from build123d import *

# Parameters (mm, degrees)
F1_DEPTH = 40


# Not quite as in the source:
# - ends of sketch curves that miss each other by under 0.0002 mm in the source are joined


with BuildPart() as f1:
    # F0 (on Front) → F1 (new body)
    with BuildSketch(Plane.XZ):
        with BuildLine():
            Line((-4.9999998882, 0), (0, 0))
            Line((0, 0), (0, 370))
            ThreePointArc((0, 370), (-25, 395), (-50, 370))
            Line((-50, 370), (-247.7872705737, 399.6680905861))
            Line((-247.7872705737, 399.6680905861), (-248.5289721923, 394.7234131282))
            Line((-248.5289721923, 394.7234131282), (-50, 364.9440672994))
            Line((-50, 364.9440672994), (-45, 364.9440672994))
            Line((-45, 364.9440672994), (-45, 370))
            ThreePointArc((-45, 370), (-25, 390), (-5, 370))
            Line((-5, 370), (-4.9999998882, 0))
        make_face()
    extrude(amount=-F1_DEPTH)


solid = f1.part
Source: CAD feature listing. Evaluate the final solid. Frame: model axes, mm. Give positions to 0.01 mm unless a question says otherwise; leave off trailing zeros. Loops run counter-clockwise (first coordinate to the right, second up) from the corner with the lowest first, then second, coordinate; pieces in that order, holes last. Notation, with made-up numbers: (1.25, 58.5) -> (20.25, 58.5) arc R10 ccw to (20.25, 71.5) -> close; hole circle Ø3 at (70.25, 62). An arc over 180 degrees is marked (long way). Use a Markdown table: item, result. Add a question column.
1) Section query B-B, the plane x = -25. Return the cut outline in (y, z).
2) Section query C-C, the plane z = 229. Return the cut outline in (x, y), then the cut area to 3 significant figures.
3) Section query A-A, the plane y = 29. Return the cut outline in (x, z).
4) First-contact query: pin 1 (1.5 mm diameter, centred on x = -47, y = 18.5, fed in from -Z); pin 2 (12 mm diameter, centred on y = 33.5, z = 296, fed in from -X); pin 3 (1 mm diameter, centred on x = -198.5, y = 6.5, fed in from +Z). Flat tips, straight axial feed; report the tip coordinate or a pass-through.
5) Pull-direction query (X, two-part tool) for faces 1 (the face through (-150.65, 19.72, 380.04)), 2 (the face through (0, 20, 182)), 3 (the face through (-147.509, 19.72, 384.626)); classes: +X half, -X half, draft (parallel to the pull), parting line (faces both ways), or undercut.
6) Line query: line 1 along X through (y, z) = (30.5, 162); line 2 along Z through (x, y) = (-59, 38); line 3 along Z through (x, y) = (-80.5, 15) (3 decimals). Output: solid intervals per line, ascending. Write a range as [from, to].
Numbers:
| question | item | result |
|---|---|---|
| 1 | outline | (0, 390) -> (40, 390) -> (40, 395) -> (0, 395) -> close |
| 2 | outline | (-5, 0) -> (0, 0) -> (0, 40) -> (-5, 40) -> close |
| 2 | area | 200 mm2 |
| 3 | outline | (-248.53, 394.72) -> (-50, 364.94) -> (-45, 364.94) -> (-45, 370) arc R20 cw to (-5, 370) -> (-5, 0) -> (0, 0) -> (0, 370) arc R25 ccw to (-50, 370) -> (-247.79, 399.67) -> close |
| 4 | pin 1 | stops at z = 364.94 |
| 4 | pin 2 | stops at x = -5 |
| 4 | pin 3 | stops at z = 392.35 |
| 5 | face 1 | -X half |
| 5 | face 2 | +X half |
| 5 | face 3 | undercut |
| 6 | line 1 | x = [-5, 0] |
| 6 | line 2 | z = [366.29, 371.35] |
| 6 | line 3 | z = [369.519, 374.575] |
